Part model, mm, in its own coordinate system. A direction names the side the tool comes from. Round coordinates to 2 decimals unless told otherwise and drop trailing zeros. Loops run counter-clockwise (first coordinate to the right, second up) from the corner with the lowest first, then second, coordinate; pieces in that order, holes last. Notation, with made-up numbers: (50.5, 24.25) -> (59.5, 24.25) arc R22 cw to (59.5, 45.25) -> close; hole circle Ø8 at (-26, 9). An arc over 180 degrees is marked (long way). Use a Markdown table: item, result. Add a question column.
Item 1: Which spindle directions (+Z, -Z, +X, -X, +Y, -Y) get a long thin tool onto all of the face, cutting with end or side? Do faces 1 (the face through (-8.39, 1, -36)), 2 (the face through (-22.125, 1, -8)), 3 (the face through (-14.1, 1.5, -16.2)). Say none if no direction does.
Item 2: Two-plate mould, pull along X, no slides. Class faces 4 (the face through (-11.185, 1.479, -8.074)), 5 (the face through (22.125, 1, -8)), 6 (the face through (17, 1, 0)): pulls with the +X half, pulls with the -X half, needs draft (parallel to the pull), parting line crosses it, or undercut.
Item 3: Probe line 1 (X direction, y = 1.4, z = -12.5); line 2 (X direction, y = 2.7, z = -10); line 3 (X direction, y = 1.5, z = -36). List the from-to ranges inside material, lowest first. Write a range as [from, to].
Item 4: Cut at A-A, the plane x = 0. List the corners of the cut face in (y, z).
Item 5: Flat gauge pins, fed straight in: pin 1 (1.5 mm diameter, centred on x = 0, y = 1.5, fed in from +Z); pin 2 (1.5 mm diameter, centred on y = 1, z = -16, fed in from -X); pin 3 (1.5 mm diameter, centred on x = 21, y = 0.5, fed in from -Z); pin 4 (1 mm diameter, centred on x = -16, z = -15.5, fed in from -Y). Where does each tip first touch, or does it go through?
Item 6: Cut at B-B, the plane z = -26.5. List the corners of the cut face in (x, y), plus the area to 3 significant figures.
```python
from build123d import *

# Parameters (mm, degrees)
BOSS_EXTRUDE1_DEPTH = 3
FILLET1_R           = 1.5
FILLET2_R           = 7
FILLET3_R           = 2


with BuildPart() as part:
    # Sketch1 → Boss-Extrude1 (new body)
    with BuildSketch(Plane(origin=(0, 0, 0), x_dir=(1, 0, 0), z_dir=(0, 1, 0))):
        with BuildLine():
            Line((-4.5, 7.94), (4.5, 7.94))
            Line((4.5, 7.94), (4.5, 0))
            Line((4.5, 0), (10.165, 0))
            Line((10.165, 0), (12.015, 14.649700441))
            ThreePointArc((12.015, 14.649700441), (14.026334206, 16.21), (15.586633764, 14.198665794))
            Line((15.586633764, 14.198665794), (13.793591523, 0))
            Line((13.793591523, 0), (22.124537234, 0))
            Line((22.124537234, 0), (22.124537234, 15.82))
            Line((22.124537234, 15.82), (25.434537234, 15.82))
            Line((25.434537234, 15.82), (28.504537234, 19.38))
            Line((28.504537234, 19.38), (29.164537234, 27.27))
            Line((29.164537234, 27.27), (32.041780145, 32.418380087))
            ThreePointArc((32.041780145, 32.418380087), (31.835, 34.03463387), (30.229008776, 34.31))
            Line((30.229008776, 34.31), (20.525, 29.416544335))
            Line((20.525, 29.416544335), (14.31, 40.08))
            Line((14.31, 40.08), (11.39, 40.08))
            Line((11.39, 40.08), (11.39, 31.5))
            ThreePointArc((11.39, 31.5), (9.89, 30), (8.39, 31.5))
            Line((8.39, 31.5), (8.39, 40.08))
            Line((8.39, 40.08), (1.5, 40.08))
            Line((1.5, 40.08), (1.5, 31.5))
            ThreePointArc((1.5, 31.5), (0, 30), (-1.5, 31.5))
            Line((-1.5, 31.5), (-1.5, 40.08))
            Line((-1.5, 40.08), (-8.39, 40.08))
            Line((-8.39, 40.08), (-8.39, 31.5))
            ThreePointArc((-8.39, 31.5), (-9.89, 30), (-11.39, 31.5))
            Line((-11.39, 31.5), (-11.39, 40.08))
            Line((-11.39, 40.08), (-14.31, 40.08))
            Line((-14.31, 40.08), (-20.525, 29.416544335))
            Line((-20.525, 29.416544335), (-30.229008776, 34.31))
            ThreePointArc((-30.229008776, 34.31), (-31.835, 34.03463387), (-32.041780145, 32.418380087))
            Line((-32.041780145, 32.418380087), (-29.164537234, 27.27))
            Line((-29.164537234, 27.27), (-28.504537234, 19.38))
            Line((-28.504537234, 19.38), (-25.434537234, 15.82))
            Line((-25.434537234, 15.82), (-22.124537234, 15.82))
            Line((-22.124537234, 15.82), (-22.124537234, 0))
            Line((-22.124537234, 0), (-13.793591523, 0))
            Line((-13.793591523, 0), (-15.586633764, 14.198665794))
            ThreePointArc((-15.586633764, 14.198665794), (-14.026334206, 16.21), (-12.015, 14.649700441))
            Line((-12.015, 14.649700441), (-10.165, 0))
            Line((-10.165, 0), (-4.5, 0))
            Line((-4.5, 0), (-4.5, 7.94))
        make_face()
    extrude(amount=BOSS_EXTRUDE1_DEPTH)

    # Fillet1
    fillet1_edges = [part.edges().sort_by_distance(p)[0] for p in [
        (4.5, 1.5, -7.94),
        (-4.5, 1.5, -7.94),
        (-10.165, 1.5, 0),
        (-22.124537234, 1.5, 0),
        (-22.124537234, 1.5, -15.82),
        (-25.434537234, 1.5, -15.82),
        (-20.525, 1.5, -29.416544335),
        (20.525, 1.5, -29.416544335),
        (25.434537234, 1.5, -15.82),
        (22.124537234, 1.5, -15.82),
        (22.124537234, 1.5, 0),
        (10.165, 1.5, 0),
    ]]
    fillet(fillet1_edges, radius=FILLET1_R)

    # Fillet2
    fillet2_edges = [part.edges().sort_by_distance(p)[0] for p in [
        (-28.504537234, 1.5, -19.38),
        (-29.164537234, 1.5, -27.27),
        (29.164537234, 1.5, -27.27),
        (28.504537234, 1.5, -19.38),
    ]]
    fillet(fillet2_edges, radius=FILLET2_R)

    # Fillet3
    fillet3_edges = [part.edges().sort_by_distance(p)[0] for p in [
        (-14.31, 1.5, -40.08),
        (14.31, 1.5, -40.08),
    ]]
    fillet(fillet3_edges, radius=FILLET3_R)


solid = part.part
```
A:
| question | item | result |
|---|---|---|
| 1 | face 1 | -Z, +Y, -Y |
| 1 | face 2 | +Z, -X, +Y, -Y |
| 1 | face 3 | +Y, -Y |
| 2 | face 4 | undercut |
| 2 | face 5 | pulls with the +X half |
| 2 | face 6 | needs draft |
| 3 | line 1 | x = [-22.12, -15.37], [-11.74, 11.74], [15.37, 22.12] |
| 3 | line 2 | x = [-22.12, -15.06], [-11.43, 11.43], [15.06, 22.12] |
| 3 | line 3 | x = [-16.69, -11.39], [-8.39, -1.5], [1.5, 8.39], [11.39, 16.69] |
| 4 | outline | (0, -30) -> (3, -30) -> (3, -7.94) -> (0, -7.94) -> close |
| 5 | pin 1 | stops at z = -7.94 |
| 5 | pin 2 | stops at x = -26.24 |
| 5 | pin 3 | stops at z = -30.16 |
| 5 | pin 4 | stops at y = 0 |
| 6 | outline | (-29.14, 0) -> (29.14, 0) -> (29.14, 3) -> (-29.14, 3) -> close |
| 6 | area | 175 mm^2 |
